Read the model definition and answer for the solid it produces. Units are mm, in the model's axes. A direction names the side the tool comes from. Coordinates: 2 decimals unless noted, no trailing zeros. Order: outer loops, then holes, each group sorted by start corner. A loop starts at its lowest first (then second) coordinate and runs counter-clockwise, first axis right, second up. Notation, with made-up numbers: (-37.75, 42.5) -> (-22.75, 42.5) arc R8 cw to (-22.75, 49.5) -> close; hole circle Ø6 at (27, 41). An arc over 180 degrees is marked (long way). Answer as a JSON object with one key per item and string values. Group by question number.
1) Consider L1, parallel to Y at x = 32.5, z = -5.25; L2, parallel to X at y = 30.5, z = -9.5; L3, parallel to X at y = 16, z = -8.5. Determine where each line is inside the solid, lowest interval first.
2) Section A-A on x = 22.5 is taken. Determine the outline of the cut face in (y, z).
3) A tool of negligible diameter and unlimited length cuts with its end or side. For faces 4 (the flat face through (9, 30, 0)), 5 (the flat face through (35, 5, 0)), from which of +Z, -Z, +X, -X, +Y, -Y can it reach the whole face along a straight path? Write none if from no direction.
4) Given pin 1 (2 mm diameter, centred on x = 33.5, y = 7.5, fed in from -Z); pin 2 (5 mm diameter, centred on x = 34, z = -4, fed in from +Y); pin 3 (1.5 mm diameter, centred on x = -5.5, y = 9, fed in from +Z), each flat-ended and moving along its own axis, determine where each tip first touches the part or whether it passes through.
5) Determine the mould class of faces 1 (the flat face through (25, 10, 2)), 2 (the flat face through (13.8, 19.86, -0.16)), 3 (the cylindrical face through (-11.523, 19.72, 0.253)) for opening direction X: released by +X, released by -X, zero draft, split by the parting line, or undercut.
6) Section C-C on y = 25 is taken. Determine the outline of the cut face in (x, z).
7) Section D-D on z = 0 is taken. Determine the outline of the cut face in (x, y).
8) Section B-B on z = -9.5 is taken. Determine the outline of the cut face in (x, y), and give its area (3 significant figures).
from build123d import *

# Parameters (mm, degrees)
BOSS_EXTRUDE1_DEPTH = 10
BOSS_EXTRUDE2_DEPTH = 20
BOSS_EXTRUDE3_DEPTH = 30


with BuildPart() as part:
    # Sketch1 → Boss-Extrude1 (new body)
    with BuildSketch(Plane(origin=(0, 0, 0), x_dir=(1, 0, 0), z_dir=(0, 1, 0))):
        with BuildLine():
            Line((0, 11.52564913), (30, 11.52564913))
            Line((30, 11.52564913), (40, -11.52564913))
            Line((40, -11.52564913), (0, -11.52564913))
            ThreePointArc((0, -11.52564913), (-11.52564913, 0), (0, 11.52564913))
        make_face()
    extrude(amount=BOSS_EXTRUDE1_DEPTH)

    # Sketch2 → Boss-Extrude2 (add)
    with BuildSketch(Plane(origin=(0, 10, 0), x_dir=(1, 0, 0), z_dir=(0, 1, 0))):
        Polygon((7.498547434, 11.52564913), (17.498547434, 11.52564913), (10, -11.52564913), (0, -11.52564913), align=None)
    extrude(amount=BOSS_EXTRUDE2_DEPTH)

    # Sketch3 → Boss-Extrude3 (add)
    with BuildSketch(Plane(origin=(0, 10, 0), x_dir=(1, 0, 0), z_dir=(0, 1, 0))):
        with BuildLine():
            Line((0, 11.52564913), (7.498547434, 11.52564913))
            Line((7.498547434, 11.52564913), (0, -11.52564913))
            ThreePointArc((0, -11.52564913), (-11.52564913, 0), (0, 11.52564913))
        make_face()
    extrude(amount=BOSS_EXTRUDE3_DEPTH)


solid = part.part
Worked answers:
{
 "1": {"L1": "y = 0 to 10", "L2": "x = -6.53 to 6.84", "L3": "x = -7.78 to 16.51"},
 "2": {"outline": "(0, -11.53) -> (10, -11.53) -> (10, 11.53) -> (0, 11.53) -> close"},
 "3": {"face 4": "+Z, +X, +Y", "face 5": "-Z, +X, +Y, -Y"},
 "4": {"pin 1": "stops at z = -5.76", "pin 2": "stops at y = 10", "pin 3": "stops at z = 10.5"},
 "5": {"face 1": "zero draft", "face 2": "released by +X", "face 3": "released by -X"},
 "6": {"outline": "(0, -11.53) -> (17.5, -11.53) -> (10, 11.53) -> (0, 11.53) arc R11.53 ccw to start"},
 "7": {"outline": "(-11.53, 0) -> (35, 0) -> (35, 10) -> (13.75, 10) -> (13.75, 30) -> (3.75, 30) -> (3.75, 40) -> (-11.53, 40) -> close"},
 "8": {"outline": "(-6.53, 0) -> (30.88, 0) -> (30.88, 10) -> (16.84, 10) -> (16.84, 30) -> (6.84, 30) -> (6.84, 40) -> (-6.53, 40) -> close", "area": "975 mm²"}
}
